from build123d import *

# Parameters (mm, degrees)
SKETCH1_R           = 2.54
BOSS_EXTRUDE1_DEPTH = 4.7625
FILLET1_R           = 6.35
CUT_EXTRUDE1_DEPTH  = 558.08584743
FILLET2_R           = 7.62


with BuildPart() as part:
    # Sketch1 → Boss-Extrude1 (new body)
    with BuildSketch(Plane.XY):
        Polygon((69.85, 0), (69.85, 57.15), (0, 57.15), (0, 508), (50.8, 508), (228.6, 50.8), (228.6, 0), align=None)
        with Locations(Location((12.7, 63.5, 0), (0, 0, 180))):
            Circle(SKETCH1_R, mode=Mode.SUBTRACT)
        with Locations(Location((38.1, 63.5, 0), (0, 0, 180))):
            Circle(SKETCH1_R, mode=Mode.SUBTRACT)
        with Locations(Location((38.1, 190.5, 0), (0, 0, 180))):
            Circle(SKETCH1_R, mode=Mode.SUBTRACT)
        with Locations(Location((12.7, 190.5, 0), (0, 0, 180))):
            Circle(SKETCH1_R, mode=Mode.SUBTRACT)
        with Locations(Location((38.1, 317.5, 0), (0, 0, 180))):
            Circle(SKETCH1_R, mode=Mode.SUBTRACT)
        with Locations(Location((12.7, 317.5, 0), (0, 0, 180))):
            Circle(SKETCH1_R, mode=Mode.SUBTRACT)
        with Locations(Location((139.7, 12.7, 0), (0, 0, 180))):
            Circle(SKETCH1_R, mode=Mode.SUBTRACT)
        with Locations(Location((139.7, 38.1, 0), (0, 0, 180))):
            Circle(SKETCH1_R, mode=Mode.SUBTRACT)
        with Locations(Location((215.9, 12.7, 0), (0, 0, 180))):
            Circle(SKETCH1_R, mode=Mode.SUBTRACT)
        with Locations(Location((215.9, 38.1, 0), (0, 0, 180))):
            Circle(SKETCH1_R, mode=Mode.SUBTRACT)
        with Locations(Location((38.1, 444.5, 0), (0, 0, 180))):
            Circle(SKETCH1_R, mode=Mode.SUBTRACT)
        with Locations(Location((12.7, 444.5, 0), (0, 0, 180))):
            Circle(SKETCH1_R, mode=Mode.SUBTRACT)
    extrude(amount=BOSS_EXTRUDE1_DEPTH)

    # Fillet1
    fillet1_edges = [part.edges().sort_by_distance(p)[0] for p in [
        (0, 508, 2.38125),
        (50.8, 508, 2.38125),
        (228.6, 50.8, 2.38125),
        (228.6, 0, 2.38125),
        (69.85, 0, 2.38125),
        (69.85, 57.15, 2.38125),
        (0, 57.15, 2.38125),
    ]]
    fillet(fillet1_edges, radius=FILLET1_R)

    # Sketch2 → Cut-Extrude1 (cut, through all)
    with BuildSketch(Plane.XY.offset(4.7625)):
        with BuildLine():
            ThreePointArc((91.574991646, 76.5566466), (99.005402277, 64.619421447), (101.6, 50.8))
            Line((101.6, 50.8), (206.797534175, 50.8))
            Line((206.797534175, 50.8), (156.422847293, 180.334909125))
            Line((156.422847293, 180.334909125), (91.574991646, 76.5566466))
        make_face()
        with BuildLine():
            ThreePointArc((50.8, 86.721024484), (62.523521168, 88.887484678), (74.342654332, 87.324606049))
            Line((74.342654332, 87.324606049), (147.2311787, 203.970628365))
            Line((147.2311787, 203.970628365), (50.8, 451.93651645))
            Line((50.8, 451.93651645), (50.8, 86.721024484))
        make_face()
    extrude(amount=-CUT_EXTRUDE1_DEPTH, mode=Mode.SUBTRACT)

    # Fillet2
    fillet2_edges = [part.edges().sort_by_distance(p)[0] for p in [
        (50.8, 86.721024484, 2.38125),
        (50.8, 451.93651645, 2.38125),
        (147.2311787, 203.970628365, 2.38125),
        (74.342654332, 87.324606049, 2.38125),
        (91.574991646, 76.5566466, 2.38125),
        (156.422847293, 180.334909125, 2.38125),
        (206.797534175, 50.8, 2.38125),
        (101.6, 50.8, 2.38125),
    ]]
    fillet(fillet2_edges, radius=FILLET2_R)


solid = part.part
Could you check a few things on this model? Use its own coordinates, in mm. A direction names the side the tool comes from. Coordinates: 2 decimals unless noted, no trailing zeros. Order: outer loops, then holes, each group sorted by start corner. A loop starts at its lowest first (then second) coordinate and runs counter-clockwise, first axis right, second up. Notation, with made-up numbers: (17.25, 52.5) - (72.25, 52.5) arc R20 cw to (72.25, 86.5) - close; hole circle Ø6 at (17.25, 24). An arc over 180 degrees is marked (long way). Answer in a Markdown table with one row per item. Add a question column.
(1) If we section it at B-B, the plane x = 115: Please give me the cut outline in (y, z).
(2) On a 3-axis mill with a long thin cutter (end or side, diameter ignored), from which of +Z, -Z, +X, -X, +Y, -Y can I reach the whole of each face in a straight line? I mean faces 4 (the face through (121.78, 124.895, 2.415)), 5 (the face through (40, 201, 4.762)). Say none if no direction works.
(3) If we mould it in two halves opening along Y, with no side actions, what happens to faces 1 (the face through (139.04, 281.1, 2.35)), 2 (the face through (182.63, 112.94, 2.41)), 3 (the face through (40, 201, 0))? For each: released by +Y, released by -Y, zero draft, split by the parting line, or undercut.
(4) If we section it at A-A, the plane y = 381.5: Please give me the cut outline in (x, z), then the cut area to 3 significant figures.
(5) I need wall thicknesses on L1, parallel to Y at x = 12.7, z = 1.2; L2, parallel to X at y = 90, z = 3.05; L3, parallel to X at y = 71, z = 4.05. Which ranges of each line are inside material? Lowest first, please.
(6) Will these pins go through, and if not, where does the flat tip stop? pin 1 (1 mm diameter, centred on x = 42.5, z = 2.5, fed in from -Y); pin 2 (2.5 mm diameter, centred on y = 38, z = 1.5, fed in from -X); pin 3 (4 mm diameter, centred on x = 38.1, y = 444.5, fed in from +Z).
(7) If we section it at C-C, the plane y = 111: Please give me the cut outline in (x, z), then the cut area to 3 significant figures.
(8) If we section it at D-D, the plane x = 25.5: Please give me the cut outline in (y, z).
Results are:
| question | item | result |
|---|---|---|
| 1 | outline | (0, 0) - (50.8, 0) - (50.8, 4.76) - (0, 4.76) - close; (114.04, 0) - (152.39, 0) - (152.39, 4.76) - (114.04, 4.76) - close; (286.85, 0) - (342.91, 0) - (342.91, 4.76) - (286.85, 4.76) - close |
| 2 | face 4 | +Z, -Z |
| 2 | face 5 | +Z, +X, -X, +Y, -Y |
| 3 | face 1 | released by +Y |
| 3 | face 2 | undercut |
| 3 | face 3 | zero draft |
| 4 | outline | (0, 0) - (50.8, 0) - (50.8, 4.76) - (0, 4.76) - close; (78.19, 0) - (99.99, 0) - (99.99, 4.76) - (78.19, 4.76) - close |
| 4 | area | 346 mm2 |
| 5 | L1 | y = 57.15 to 60.96, 66.04 to 187.96, 193.04 to 314.96, 320.04 to 441.96, 447.04 to 508 |
| 5 | L2 | x = 0 to 54.04, 75.51 to 99.98, 191.55 to 213.36 |
| 5 | L3 | x = 0 to 95.8, 198.94 to 220.74 |
| 6 | pin 1 | stops at y = 57.15 |
| 6 | pin 2 | stops at x = 69.85 |
| 6 | pin 3 | passes through |
| 7 | outline | (0, 0) - (50.8, 0) - (50.8, 4.76) - (0, 4.76) - close; (89.14, 0) - (113.1, 0) - (113.1, 4.76) - (89.14, 4.76) - close; (183.39, 0) - (205.19, 0) - (205.19, 4.76) - (183.39, 4.76) - close |
| 7 | area | 460 mm2 |
| 8 | outline | (57.15, 0) - (508, 0) - (508, 4.76) - (57.15, 4.76) - close |
